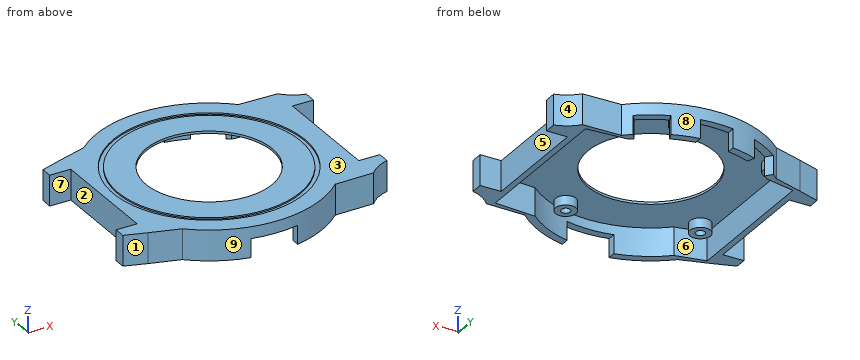
```python
from build123d import *

# Parameters (mm, degrees)
PAD_DEPTH       = 6.5
POCKET_DEPTH    = 6
SKETCH002_R     = 13.5
POCKET001_DEPTH = 1
SKETCH003_W     = 5.4
SKETCH003_H     = 6.5
PAD001_DEPTH    = 4.5
POCKET002_DEPTH = 10
SKETCH010_W     = 3.95
SKETCH010_H     = 6.5
PAD002_DEPTH    = 4.5
POCKET005_DEPTH = 10
SKETCH012_R     = 0.6
POCKET006_DEPTH = 2
SKETCH014_R     = 20.45
SKETCH014_R_2   = 19.5
POCKET008_DEPTH = 0.3
SKETCH015_R     = 2.2
SKETCH015_R_2   = 0.975
PAD003_DEPTH    = 2
POCKET009_DEPTH = 4
POCKET010_DEPTH = 4


with BuildPart() as part:
    # Sketch → Pad (new body)
    with BuildSketch(Plane.XY):
        with BuildLine():
            Line((-22.5019915649, 16), (-22.5019915649, -16))
            Line((-22.5019915649, -16), (-16.2858834577, -17.9000000001))
            ThreePointArc((-16.2858834577, -17.9000000001), (0.2206895737, -24.1989937004), (16.6096357576, -17.5999999999))
            Line((16.6096357576, -17.5999999999), (24.9082802252, -17.45))
            Line((24.9082802252, 17.45), (24.9082802252, -17.45))
            Line((16.6096357576, 17.6), (24.9082802252, 17.45))
            ThreePointArc((16.6096357576, 17.6), (0.2206895736, 24.1989937004), (-16.2858834578, 17.9))
            Line((-22.5019915649, 16), (-16.2858834578, 17.9))
        make_face()
    extrude(amount=PAD_DEPTH)

    # Sketch001 → Pocket (cut)
    with BuildSketch(Plane.XY):
        with BuildLine():
            Line((-14.8539557021, 16.9), (-21.2122180433, 15.55))
            Line((-21.2122180433, 15.55), (-21.2122180433, -15.55))
            Line((-21.2122180433, -15.55), (-14.8539557021, -16.9))
            ThreePointArc((-14.8539557021, -16.9), (-0.0760301383, -22.4998715423), (14.739402973, -17))
            Line((14.739402973, -17), (23.6191552218, -16.4))
            Line((23.6191552218, 16.4), (23.6191552218, -16.4))
            Line((14.739402973, 17), (23.6191552218, 16.4))
            ThreePointArc((14.739402973, 17), (-0.0760301383, 22.4998715423), (-14.8539557021, 16.9))
        make_face()
    extrude(amount=POCKET_DEPTH, mode=Mode.SUBTRACT)

    # Sketch002 (on Face19 of Pocket) → Pocket001 (cut)
    with BuildSketch(Plane(origin=(0, 0, 6), x_dir=(1, 0, 0), z_dir=(0, 0, -1))):
        Circle(SKETCH002_R)
    extrude(amount=-POCKET001_DEPTH, mode=Mode.SUBTRACT)

    # Sketch003 (on Face7 of Pad) → Pad001 (join)
    with BuildSketch(Plane.YZ.offset(24.9082802252)):
        with Locations((-14.75, 3.25)):
            Rectangle(SKETCH003_W, SKETCH003_H)
        with Locations((14.75, 3.25)):
            Rectangle(SKETCH003_W, SKETCH003_H)
    extrude(amount=PAD001_DEPTH)

    # Sketch006 (on Face22 of Pad001) → Pocket002 (cut)
    with BuildSketch(Plane.XY.offset(6.5)):
        with BuildLine():
            ThreePointArc((24.9082802252, 17.45), (26.9423471239, 15.7065020586), (29.4082802252, 14.6594169811))
            Line((29.4082802252, 17.45), (29.4082802252, 14.6594169811))
            Line((29.4082802252, 17.45), (24.9082802252, 17.45))
        make_face()
        with BuildLine():
            ThreePointArc((29.4082802252, -14.6594169811), (26.9423471239, -15.7065020586), (24.9082802252, -17.45))
            Line((29.4082802252, -17.45), (24.9082802252, -17.45))
            Line((29.4082802252, -14.6594169811), (29.4082802252, -17.45))
        make_face()
    extrude(amount=-POCKET002_DEPTH, mode=Mode.SUBTRACT)

    # Sketch010 (on Face3 of Pad) → Pad002 (join)
    with BuildSketch(Plane(origin=(-22.5019915649, 0, 0), x_dir=(0, -1, 0), z_dir=(-1, 0, 0))):
        with Locations((-14.025, 3.25)):
            Rectangle(SKETCH010_W, SKETCH010_H)
        with Locations((14.025, 3.25)):
            Rectangle(SKETCH010_W, SKETCH010_H)
    extrude(amount=PAD002_DEPTH)

    # Sketch011 (on Face28 of Pad002) → Pocket005 (cut)
    with BuildSketch(Plane.XY.offset(6.5)):
        Polygon((-27.0019915649, 16), (-22.5019915649, 16), (-27.0019915649, 14.5), align=None)
        Polygon((-22.5019915649, -16), (-27.0019915649, -14.5), (-27.0019915649, -16), align=None)
    extrude(amount=-POCKET005_DEPTH, mode=Mode.SUBTRACT)

    # Sketch012 (on Face23 of Pocket005) → Pocket006 (cut)
    with BuildSketch(Plane(origin=(23.6191552218, 0, 0), x_dir=(0, -1, 0), z_dir=(-1, 0, 0))):
        with Locations((12.9594169811, 8.2)):
            Circle(SKETCH012_R)
    extrude(amount=-POCKET006_DEPTH, mode=Mode.SUBTRACT)

    # Sketch014 (on Face10 of Pad) → Pocket008 (cut)
    with BuildSketch(Plane.XY.offset(6.5)):
        Circle(SKETCH014_R)
        Circle(SKETCH014_R_2, mode=Mode.SUBTRACT)
    extrude(amount=-POCKET008_DEPTH, mode=Mode.SUBTRACT)

    # Sketch015 (on Face19 of Pocket) → Pad003 (join)
    with BuildSketch(Plane(origin=(0, 0, 6), x_dir=(1, 0, 0), z_dir=(0, 0, -1))):
        with Locations((-18.42, 13.32)):
            Circle(SKETCH015_R)
        with Locations((-18.42, 13.32)):
            Circle(SKETCH015_R_2, mode=Mode.SUBTRACT)
        with Locations((7.27, 18.56)):
            Circle(SKETCH015_R)
        with Locations((7.27, 18.56)):
            Circle(SKETCH015_R_2, mode=Mode.SUBTRACT)
        with Locations((5.37, -19.79)):
            Circle(SKETCH015_R)
        with Locations((5.37, -19.79)):
            Circle(SKETCH015_R_2, mode=Mode.SUBTRACT)
        with Locations((-18.42, -13.32)):
            Circle(SKETCH015_R)
        with Locations((-18.42, -13.32)):
            Circle(SKETCH015_R_2, mode=Mode.SUBTRACT)
    extrude(amount=PAD003_DEPTH)

    # Sketch016 → Pocket009 (cut)
    with BuildSketch(Plane(origin=(0, 0, 0), x_dir=(-1, 0, 0), z_dir=(0, 0, 1))):
        with BuildLine():
            Line((-5, 23.6778377391), (-5, 21.9374109685))
            ThreePointArc((5, 21.9374109685), (0, 22.5), (-5, 21.9374109685))
            Line((5, 23.6778377391), (5, 21.9374109685))
            ThreePointArc((5, 23.6778377391), (0, 24.2), (-5, 23.6778377391))
        make_face()
    extrude(amount=POCKET009_DEPTH, mode=Mode.SUBTRACT)

    # Sketch017 → Pocket010 (cut)
    with BuildSketch(Plane(origin=(0, 0, 0), x_dir=(-1, 0, 0), z_dir=(0, 0, 1))):
        with BuildLine():
            Line((-3.499984119, -22.2261132717), (-3.5, -23.9455632634))
            ThreePointArc((-3.5, -23.9455632634), (0, -24.2000019575), (3.5, -23.9455632634))
            Line((3.5000158811, -22.2261082701), (3.5, -23.9455632634))
            ThreePointArc((-3.499984119, -22.2261132717), (1.60767e-05, -22.5), (3.5000158811, -22.2261082701))
        make_face()
        with BuildLine():
            ThreePointArc((-13.9498796389, -17.6536358312), (-11.25, -19.4855715851), (-8.3135572795, -20.9077680626))
            Line((-8.3135572795, -20.9077680626), (-8.9416927184, -22.487466094))
            ThreePointArc((-15.0038705449, -18.987466094), (-12.1, -20.9578147716), (-8.9416927184, -22.487466094))
            Line((-13.9498796389, -17.6536358312), (-15.0038705449, -18.987466094))
        make_face()
        with BuildLine():
            ThreePointArc((8.3135572795, -20.9077680626), (11.25, -19.4855715851), (13.9498796389, -17.6536358312))
            Line((13.9498796389, -17.6536358312), (15.0038705449, -18.987466094))
            ThreePointArc((8.9416927184, -22.487466094), (12.1, -20.9578147716), (15.0038705449, -18.987466094))
            Line((8.3135572795, -20.9077680626), (8.9416927184, -22.487466094))
        make_face()
    extrude(amount=POCKET010_DEPTH, mode=Mode.SUBTRACT)


solid = part.part
```
Geometry: final body of the model. Coordinates: model frame, mm. Face numbers are marked on the shaded views. A direction names the side the tool comes from. Give positions to 0.01 mm unless a question says otherwise; leave off trailing zeros. Loops run counter-clockwise (first coordinate to the right, second up) from the corner with the lowest first, then second, coordinate; pieces in that order, holes last. Notation, with made-up numbers: (78.25, 59.25) -> (119.25, 59.25) arc R33 cw to (119.25, 91.25) -> close; hole circle Ø7 at (80, -25). An arc over 180 degrees is marked (long way). Use one line per item in the form item = value.
Item 1: Section query A-A on x = 0. Output: boundary loops of the cut face in (y, z).
A:
outline = (-24.2, 4) -> (-22.5, 4) -> (-22.5, 6) -> (-13.5, 6) -> (-13.5, 6.5) -> (-19.5, 6.5) -> (-19.5, 6.2) -> (-20.45, 6.2) -> (-20.45, 6.5) -> (-24.2, 6.5) -> close; (13.5, 6) -> (22.5, 6) -> (22.5, 4) -> (24.2, 4) -> (24.2, 6.5) -> (20.45, 6.5) -> (20.45, 6.2) -> (19.5, 6.2) -> (19.5, 6.5) -> (13.5, 6.5) -> close
Item 2: Line query: probe 1 along Y at (x, z) = (0, 6.4); probe 2 along X at (y, z) = (3, 1.25); probe 3 along X at (y, z) = (-13.5, 0.5). Output: solid intervals per line, ascending.
A:
probe_1 = -24.2 to -20.45, -19.5 to -13.5, 13.5 to 19.5, 20.45 to 24.2
probe_2 = -22.5 to -21.21, 23.62 to 24.91
probe_3 = -27 to -21.21, 23.62 to 29.41
Item 3: Section query D-D on z = 1.75. Give the number of separate pieces and of enclosed holes in the cut face, and give its area (3 significant figures).
A:
separate_pieces = 4
enclosed_holes = 0
area = 239 mm^2
Item 4: Access query for the marked faces 5, 6, 7, 8 and 9. Directions: +Z, -Z, +X, -X, +Y, -Y. A direction counts if a zero-diameter tool reaches every point of the face in a straight line with its end or side. Return the directions, or none.
A:
face_5 = +Z, -Z, +X
face_6 = -Z
face_7 = +Z, -Z, -X
face_8 = +Z, -Z, +Y
face_9 = +Z, -Z, -Y
Item 5: Draft query along Y for the marked faces 1, 2, 3 and 4. Return one class per face: pulls with the +Y half, pulls with the -Y half, needs draft (parallel to the pull), parting line crosses it, or undercut.
A:
face_1 = pulls with the -Y half
face_2 = undercut
face_3 = needs draft
face_4 = pulls with the +Y half
Item 6: Section query B-B on y = -8.5. Output: boundary loops of the cut face in (x, z), and give its area (3 significant figures).
A:
outline = (-22.5, 0) -> (-21.21, 0) -> (-21.21, 6) -> (-10.49, 6) -> (-10.49, 6.5) -> (-17.55, 6.5) -> (-17.55, 6.2) -> (-18.6, 6.2) -> (-18.6, 6.5) -> (-22.5, 6.5) -> close; (10.49, 6) -> (23.62, 6) -> (23.62, 0) -> (24.91, 0) -> (24.91, 6.5) -> (18.6, 6.5) -> (18.6, 6.2) -> (17.55, 6.2) -> (17.55, 6.5) -> (10.49, 6.5) -> close
area = 28.1 mm^2
Item 7: Pin query (flat end, axial travel): P1, Ø3, axis at x = 12.5, z = 1, coming from the -Y side; P2, Ø12, axis at x = -8.5, y = 13, coming from the -Z side; P3, Ø2, axis at x = 7, y = -19, coming from the -Z side. Return the tip coordinate at first contact, or that it passes through.
A:
P1 = -21.56
P2 = 6
P3 = 4
